Job drawing, mm, ordinate dimensions from the low corner. One solid piece. A direction names the side the tool comes from. Give positions to 0.01 mm unless a question says otherwise; leave off trailing zeros. Loops run counter-clockwise (first coordinate to the right, second up) from the corner with the lowest first, then second, coordinate; pieces in that order, holes last. Notation, with made-up numbers: (79.25, 14.5) -> (135.25, 14.5) arc R16 ccw to (135.25, 25.5) -> close; hole circle Ø3 at (24.5, 28). An arc over 180 degrees is marked (long way). Answer as a JSON object with one key per item and string values. Group by question number.
Q1. Band-saw the part on C-C, the plane y = 24.5. Write the cut outline in (x, z).
Q2. Band-saw the part on D-D, the plane z = 42. Write the cut outline in (x, y), plus the area to 3 significant figures.
Q3. Wall check: probe 1 along Z at (x, y) = (24.5, 19.5); probe 2 along Y at (x, z) = (7, 2); probe 3 along Y at (x, z) = (2, 41). Give the ranges that are in metal, low to high. Write a range as from..to.
Q4. Band-saw the part on A-A, the plane x = 18. Write the cut outline in (y, z), plus the area to 3 significant figures.
Q5. Tool access for the marked faces 4, 5 and 6: list every direction of +Z, -Z, +X, -X, +Y, -Y with a clear straight run to the whole face (end or side of a thin tool).
Q6. Band-saw the part on B-B, the plane z = 8.25. Write the cut outline in (x, y).
Q7. Two-plate mould, pull along X, no slides. Class the marked faces 1, 2 and 3: pulls with the +X half, pulls with the -X half, needs draft (parallel to the pull), parting line crosses it, or undercut.
Q8. Drop flat-ended pins along their axis: pin 1 (3.5 mm diameter, centred on y = 20.5, z = 8.5, fed in from +X); pin 2 (3 mm diameter, centred on x = 1, y = 19.5, fed in from -Z); pin 3 (9.5 mm diameter, centred on x = 15, y = 22, fed in from +Z); pin 4 (12 mm diameter, centred on x = 17.5, y = 18, fed in from +Z). Give the stop position or say it passes through.
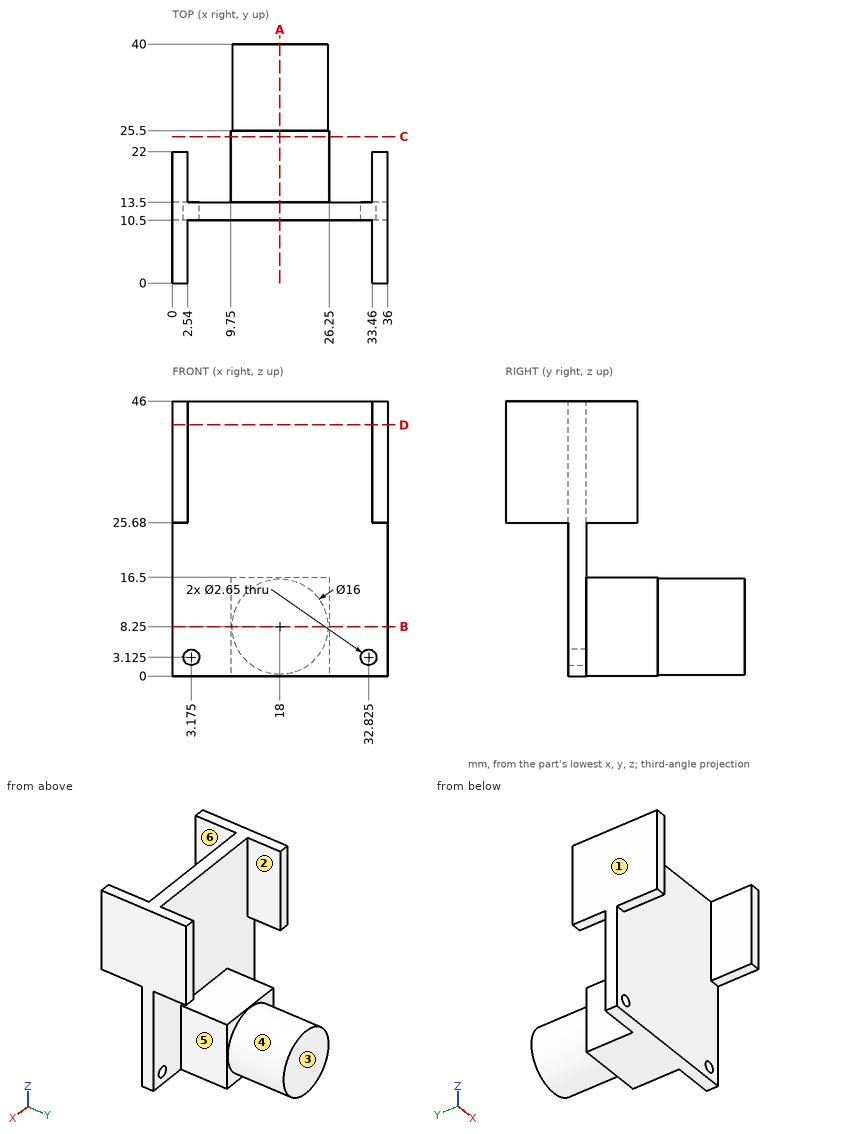
Worked answers:
{
 "1": {"outline": "(9.75, 0) -> (26.25, 0) -> (26.25, 16.5) -> (9.75, 16.5) -> close"},
 "2": {"outline": "(0, 0) -> (2.54, 0) -> (2.54, 10.5) -> (33.46, 10.5) -> (33.46, 0) -> (36, 0) -> (36, 22) -> (33.46, 22) -> (33.46, 13.5) -> (2.54, 13.5) -> (2.54, 22) -> (0, 22) -> close", "area": "205 mm2"},
 "3": {"probe 1": "0..16.5", "probe 2": "10.5..13.5", "probe 3": "0..22"},
 "4": {"outline": "(10.5, 0) -> (25.5, 0) -> (25.5, 0.25) -> (40, 0.25) -> (40, 16.25) -> (25.5, 16.25) -> (25.5, 16.5) -> (13.5, 16.5) -> (13.5, 46) -> (10.5, 46) -> close", "area": "568 mm2"},
 "5": {"face 4": "+Y", "face 5": "+Z, -Z, +X, +Y", "face 6": "+Z, -Z, -Y"},
 "6": {"outline": "(0, 10.5) -> (36, 10.5) -> (36, 13.5) -> (26.25, 13.5) -> (26.25, 25.5) -> (26, 25.5) -> (26, 40) -> (10, 40) -> (10, 25.5) -> (9.75, 25.5) -> (9.75, 13.5) -> (0, 13.5) -> close"},
 "7": {"face 1": "pulls with the -X half", "face 2": "undercut", "face 3": "needs draft"},
 "8": {"pin 1": "x = 26.25", "pin 2": "z = 25.68", "pin 3": "z = 16.5", "pin 4": "z = 46"}
}
